Here's how the part is built. I have some questions about the finished solid (model axes, mm). Face numbers are marked on the shaded views. A direction names the side the tool comes from. Give positions to 0.01 mm unless a question says otherwise; leave off trailing zeros. Write each loop counter-clockwise with the first axis right and the second up, starting at its lowest first coordinate (ties: lowest second). Pieces come first, ordered by that corner, then holes. Notation, with made-up numbers: (48.5, -2.5) - (107.5, -2.5) arc R36 cw to (107.5, 31.5) - close; hole circle Ø4 at (61.5, 21). An arc over 180 degrees is marked (long way). Use a Markdown table: item, result.
```python
from build123d import *

# Parameters (mm, degrees)
SKETCH3_R           = 14.9225
BOSS_EXTRUDE1_DEPTH = 9.525
SKETCH11_R          = 2.38125
CUT_EXTRUDE3_DEPTH  = 6.35
SKETCH12_R          = 7.9375
SKETCH12_R_2        = 5.715
CUT_EXTRUDE4_DEPTH  = 1.27
THREAD1_PITCH       = 1.5875
CUT_EXTRUDE5_START  = -6.35
SKETCH13_R          = 2.38125
CUT_EXTRUDE5_DEPTH  = 6.35
CUT_EXTRUDE6_START  = -4.7625
SKETCH14_R          = 14.9225
CUT_EXTRUDE6_DEPTH  = 4.7625


with BuildPart() as part:
    # Sketch3 → Boss-Extrude1 (new body)
    with BuildSketch(Plane.XY):
        with Locations((8.347593151, 27.723781851)):
            Circle(SKETCH3_R)
    extrude(amount=-BOSS_EXTRUDE1_DEPTH)

    # Sketch11 → Cut-Extrude3 (cut)
    with BuildSketch(Plane.XY):
        with Locations((8.347593151, 27.723781851)):
            Circle(SKETCH11_R)
    extrude(amount=-CUT_EXTRUDE3_DEPTH, mode=Mode.SUBTRACT)

    # Sketch12 → Cut-Extrude4 (cut)
    with BuildSketch(Plane.XY):
        with Locations((8.347593151, 27.723781851)):
            Circle(SKETCH12_R)
        with Locations((8.347593151, 27.723781851)):
            Circle(SKETCH12_R_2, mode=Mode.SUBTRACT)
    extrude(amount=-CUT_EXTRUDE4_DEPTH, mode=Mode.SUBTRACT)

    # Thread1: the profile of Thread Profile1 profile screwed along a right-hand helix of 4.8 turns, 8 arcs to a turn; built about Z, then put on its axis
    thread1_z = Axis((0, 0, 0), (0, 0, 1))
    thread1_corners = [(14.9228, 0, -0.000173205), (14.9228, 0, 0.694704453), (14.492870212, 0, 0.446484374), (14.492870212, 0, 0.248046874)]
    with BuildLine(mode=Mode.PRIVATE) as thread1_profile:
        Line(thread1_corners[0], thread1_corners[1])
        Line(thread1_corners[1], thread1_corners[2])
        Line(thread1_corners[2], thread1_corners[3])
        Line(thread1_corners[3], thread1_corners[0])
    thread1_cap = Face(thread1_profile.wire())
    thread1_turn_angles = [0, 22.5, 45, 67.5, 90, 112.5, 135, 157.5, 180, 202.5, 225, 247.5, 270, 292.5, 315, 337.5, 360]
    thread1_turn_weights = [1, 0.9238795325112867, 1, 0.9238795325112867, 1, 0.9238795325112867, 1, 0.9238795325112867, 1, 0.9238795325112867, 1, 0.9238795325112867, 1, 0.9238795325112867, 1, 0.9238795325112867, 1]
    thread1_turn_rails = [Edge.make_bspline([Vector(p[0], p[1], 0).rotate(thread1_z, thread1_turn_angles[k]) / thread1_turn_weights[k] + Vector(0, 0, p[2] + THREAD1_PITCH * thread1_turn_angles[k] / 360) for k in range(17)], [0, 0, 0, 1, 1, 2, 2, 3, 3, 4, 4, 5, 5, 6, 6, 7, 7, 8, 8, 8], 2, thread1_turn_weights) for p in thread1_corners]
    thread1_turn_sides = [Face.make_surface_from_curves(thread1_turn_rails[p[0]], thread1_turn_rails[p[1]]) for p in [(0, 1), (1, 2), (2, 3), (3, 0)]]
    thread1_last_angles = [1440, 1462.5, 1485, 1507.5, 1530, 1552.5, 1575, 1597.5, 1620, 1642.5, 1665, 1687.5, 1710, 1719, 1728]
    thread1_last_weights = [1, 0.9238795325112867, 1, 0.9238795325112867, 1, 0.9238795325112867, 1, 0.9238795325112867, 1, 0.9238795325112867, 1, 0.9238795325112867, 1, 0.9876883405951378, 1]
    thread1_last_rails = [Edge.make_bspline([Vector(p[0], p[1], 0).rotate(thread1_z, thread1_last_angles[k]) / thread1_last_weights[k] + Vector(0, 0, p[2] + THREAD1_PITCH * thread1_last_angles[k] / 360) for k in range(15)], [0, 0, 0, 1, 1, 2, 2, 3, 3, 4, 4, 5, 5, 6, 6, 7, 7, 7], 2, thread1_last_weights) for p in thread1_corners]
    thread1_last_sides = [Face.make_surface_from_curves(thread1_last_rails[p[0]], thread1_last_rails[p[1]]) for p in [(0, 1), (1, 2), (2, 3), (3, 0)]]
    thread1 = Plane(origin=(8.347593151, 27.723781851, 0.79375), x_dir=(-1, 0, 0), z_dir=(0, 0, -1)) * Solid(Shell([*[p.moved(Location((0, 0, THREAD1_PITCH * i))) for i in range(4) for p in thread1_turn_sides], *thread1_last_sides, thread1_cap, thread1_cap.rotate(thread1_z, 1728).moved(Location((0, 0, THREAD1_PITCH * 1728 / 360)))]))
    add(thread1, mode=Mode.SUBTRACT)

    # Sketch13 → Cut-Extrude5 (cut)
    with BuildSketch(Plane(origin=(0, 0, -9.525), x_dir=(-1, 0, 0), z_dir=(0, 0, -1)).offset(CUT_EXTRUDE5_START)):
        with Locations(Location((-8.347593151, 27.723781851, 0), (0, 0, 180))):
            Circle(SKETCH13_R)
    extrude(amount=CUT_EXTRUDE5_DEPTH, mode=Mode.SUBTRACT)

    # Sketch14 → Cut-Extrude6 (cut)
    with BuildSketch(Plane(origin=(0, 0, -9.525), x_dir=(-1, 0, 0), z_dir=(0, 0, -1)).offset(CUT_EXTRUDE6_START)):
        with Locations((-8.347593151, 27.723781851)):
            Circle(SKETCH14_R)
        Polygon((1.186658464, 22.240576024), (1.168128197, 33.239083042), (-8.366123418, 38.722288869), (-17.881844766, 33.206987678), (-17.863314499, 22.20848066), (-8.329062884, 16.725274833), align=None, mode=Mode.SUBTRACT)
    extrude(amount=CUT_EXTRUDE6_DEPTH, mode=Mode.SUBTRACT)


solid = part.part
```
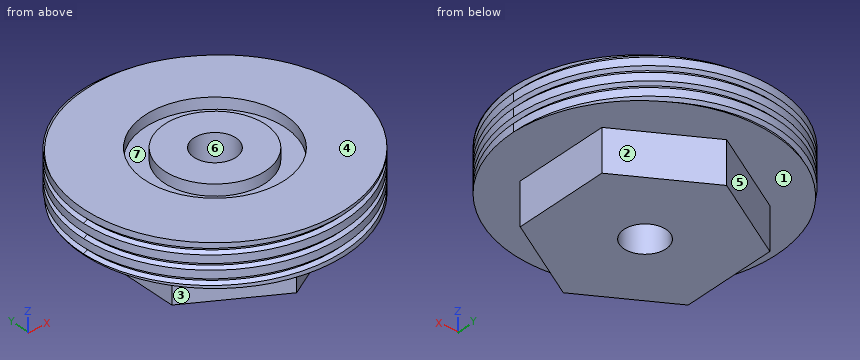
Item 1: For the marked faces 1, 2 and 3, which set-ups out of +Z, -Z, +X, -X, +Y, -Y let a thin tool reach every point of the face, with its end or its side?
Values:
| item | result |
|---|---|
| face 1 | -Z |
| face 2 | -Z, +X, +Y |
| face 3 | -Z, -X, -Y |
Item 2: If we section it at A-A, the plane z = -6.5: Write out the boundary of the cut face in (x, y).
Values:
| item | result |
|---|---|
| outline | (-1.19, 22.24) - (8.33, 16.73) - (17.86, 22.21) - (17.88, 33.21) - (8.37, 38.72) - (-1.17, 33.24) - close; hole circle Ø4.76 at (8.35, 27.72) |
Item 3: Will these pins go through, and if not, where does the flat tip stop? pin 1 Ø6 at (x, y) = (16.5, 28) entering from +Z; pin 2 Ø1.5 at (y, z) = (34.5, -1.5) entering from +X; pin 3 Ø1 at (x, z) = (19, -4.5) entering from +Y; pin 4 Ø1.5 at (y, z) = (20.5, -4) entering from -X.
Values:
| item | result |
|---|---|
| pin 1 | stops at z = 0 |
| pin 2 | stops at x = 22 |
| pin 3 | stops at y = 38.66 |
| pin 4 | stops at x = -5.09 |
Item 4: I need wall thicknesses on line 1 along Z through (x, y) = (15.25, 40.75); line 2 along Z through (x, y) = (2.5, 33) (3 decimals); line 3 along Y through (x, z) = (7.75, -0.5). Which ranges of each line are inside material? Lowest first, please. Write a range as [from, to].
Values:
| item | result |
|---|---|
| line 1 | z = [-4.59, -3.49], [-3.01, -1.9], [-1.42, -0.32] |
| line 2 | z = [-9.525, -1.27] |
| line 3 | y = [12.98, 19.81], [22.04, 25.42], [30.03, 33.41], [35.64, 42.63] |
Item 5: Thinking about a two-plate mould opening in X: for the marked faces 4, 5, 6 and 7, which applies, +X half, -X half, draft (parallel to the pull), parting line (faces both ways), or undercut?
Values:
| item | result |
|---|---|
| face 4 | draft |
| face 5 | -X half |
| face 6 | undercut |
| face 7 | undercut |
